Solid Edge part; units mm, degrees
sketch "Sketch1" plane through (0, 0, 0) normal (0, 0, 1) x (1, 0, 0)
  line L0 (-49.925, -25) -> (49.925, -25)
  line L1 (49.925, -25) -> (49.925, 25)
  line L2 (49.925, 25) -> (-49.925, 25)
  line L3 (-49.925, 25) -> (-49.925, -25)
extrude "Protrusion1" add sketch "Sketch1" against normal blind 20
sketch "Sketch2" plane through (0, 0, 0) normal (0, 0, 1) x (1, 0, 0)
  line L0 (-49.925, 25) -> (-12, 25)
  line L1 (-12, 25) -> (-12, 8)
  line L2 (-12, 8) -> (-49.925, 8)
  line L3 (-49.925, 8) -> (-49.925, 25)
  line L4 (49.925, 25) -> (12, 25)
  line L5 (12, 25) -> (12, 8)
  line L6 (12, 8) -> (49.925, 8)
  line L7 (49.925, 8) -> (49.925, 25)
extrude "ExtrudedCutout_1" cut sketch "Sketch2" against normal blind 20
sketch "Sketch3" plane through (0, 0, 0) normal (0, 0, 1) x (1, 0, 0)
  arc A0 (-49.925, -5) -> (-12, 8) centre (-49.166, 54.6052) ccw
  line L0 (-49.925, 8) -> (-12, 8)
  line L1 (-49.925, -5) -> (-49.925, 8)
  arc A1 (49.925, -5) -> (12, 8) centre (49.166, 54.6052) cw
  line L2 (12, 8) -> (49.925, 8)
  line L3 (49.925, 8) -> (49.925, -5)
extrude "ExtrudedCutout_2" cut sketch "Sketch3" against normal blind 20
fillet "Round_1" radius 10 4 edges at (49.925, -25, -10) (49.925, -5, -10) (-49.925, -25, -10) (-49.925, -5, -10)
Source: CAD feature listing. Evaluate the final solid. Frame: model axes, mm. A direction names the side the tool comes from. Give positions to 0.01 mm unless a question says otherwise; leave off trailing zeros. Write each loop counter-clockwise with the first axis right and the second up, starting at its lowest first coordinate (ties: lowest second). Pieces come first, ordered by that corner, then holes. Notation, with made-up numbers: (48.5, -1) -> (90.5, -1) arc R24 cw to (90.5, 27) -> close; hole circle Ø11 at (-31, 21.5). An arc over 180 degrees is marked (long way). Return JSON: item names as keys, results as strings. Group by question number.
1. Section C-C, the plane x = -26. Output: boundary loops of the cut face in (y, z).
2. Material intervals for line 1 (X direction, y = 19.5, z = -15); line 2 (Y direction, x = 16, z = -14); line 3 (X direction, y = -16, z = -11.5), sorted ascending. Write a range as from..to.
3. Access query for faces 1 (the face through (-1, -25, -10)), 2 (the face through (12, 17, -10)), 3 (the face through (-12, 17, -10)). Directions: +Z, -Z, +X, -X, +Y, -Y. A direction counts if a zero-diameter tool reaches every point of the face in a straight line with its end or side. Return the directions, or none.
4. Pin query (flat end, axial travel): pin 1 Ø5 at (y, z) = (17, -6.5) entering from -X; pin 2 Ø1.5 at (y, z) = (4, -16.5) entering from +X; pin 3 Ø5 at (y, z) = (-9, -14) entering from +X. Return the tip coordinate at first contact, or that it passes through.
5. Section B-B, the plane y = 15. Output: boundary loops of the cut face in (x, z), then the cut area to 3 significant figures.
6. Section A-A, the plane z = -9. Output: boundary loops of the cut face in (x, y) (3 decimals).
Determined:
{
 "1": {"outline": "(-25, -20) -> (-0.32, -20) -> (-0.32, 0) -> (-25, 0) -> close"},
 "2": {"line 1": "x = -12..12", "line 2": "y = -25..5.07", "line 3": "x = -49.87..49.87"},
 "3": {"face 1": "+Z, -Z, +X, -X, -Y", "face 2": "+Z, -Z, +X, +Y", "face 3": "+Z, -Z, -X, +Y"},
 "4": {"pin 1": "stops at x = -12", "pin 2": "stops at x = 18.9", "pin 3": "stops at x = 49.5"},
 "5": {"outline": "(-12, -20) -> (12, -20) -> (12, 0) -> (-12, 0) -> close", "area": "480 mm2"},
 "6": {"outline": "(-49.925, -15) arc R10 ccw to (-39.925, -25) -> (39.925, -25) arc R10 ccw to (49.925, -15) -> (49.925, -14.389) arc R10 ccw to (41.253, -4.477) arc R59.61 cw to (12, 8) -> (12, 25) -> (-12, 25) -> (-12, 8) arc R59.61 cw to (-41.253, -4.477) arc R10 ccw to (-49.925, -14.389) -> close"}
}
